Geometry: see drawing. Coordinates: mm, zero at the bounding-box minimum. A direction names the side the tool comes from. Give positions to 0.01 mm unless a question says otherwise; leave off trailing zeros. Write each loop counter-clockwise with the first axis right and the second up, starting at its lowest first coordinate (ties: lowest second). Pieces come first, ordered by that corner, then holes. Notation, with made-up numbers: (66, -11.5) -> (111, -11.5) arc R25 ccw to (111, 18.5) -> close; hole circle Ø1 at (-36, -17.5). An arc over 180 degrees is marked (long way). Use CSV: the item, a comma, the result in double quotes. Start each with the question number.
1) Contact query for flat-ended pins moving along their axis: P1, Ø5, axis at y = 376.5, z = 3.5, coming from the -X side; P2, Ø6, axis at x = 2, z = 17, coming from the +Y side; P3, Ø1, axis at x = 13, y = 163, coming from the -Z side; P4, Ø8, axis at y = 96.5, z = 5, coming from the +X side. Output: stop coordinate, or through.
2) Section A-A (z = 12.5). Output: boundary loops of the cut face in (x, y), plus the area to 3 significant figures.
3) Section B-B (y = 82). Output: boundary loops of the cut face in (x, z), plus the area to 3 significant figures.
4) Material intervals for line 1 (Y direction, x = 14.5, z = 11.75); line 2 (X direction, y = 422, z = 15); line 3 (Y direction, x = 18.75, z = 17) (1 decimal), sorted ascending. Write a range as [from, to].
5) Set-up query: the marked faces 1, 2 and 3. Return all of +Z, -Z, +X, -X, +Y, -Y with unobstructed straight access to the full face (end or side cutting, diameter ignored); none if empty.
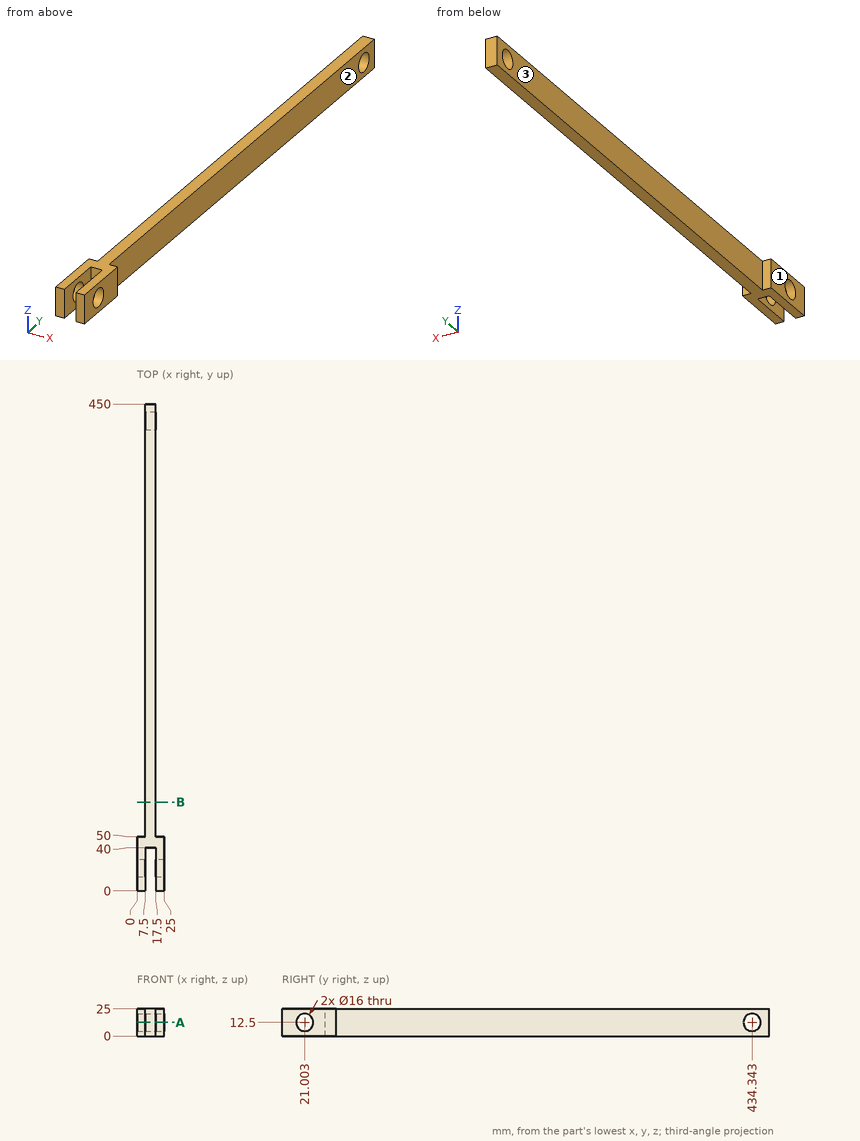
Answers follow:
1,P1,"stops at x = 7.5"
1,P2,"stops at y = 50"
1,P3,"stops at z = 0"
1,P4,"stops at x = 17.5"
2,outline,"(0, 0) -> (7.5, 0) -> (7.5, 13) -> (0, 13) -> close; (0, 29) -> (7.5, 29) -> (7.5, 40) -> (17.5, 40) -> (17.5, 29) -> (25, 29) -> (25, 50) -> (17.5, 50) -> (17.5, 426.34) -> (7.5, 426.34) -> (7.5, 50) -> (0, 50) -> close; (7.5, 442.34) -> (17.5, 442.34) -> (17.5, 450) -> (7.5, 450) -> close; (17.5, 0) -> (25, 0) -> (25, 13) -> (17.5, 13) -> close"
2,area,"4,450 mm^2"
3,outline,"(7.5, 0) -> (17.5, 0) -> (17.5, 25) -> (7.5, 25) -> close"
3,area,"250 mm^2"
4,line 1,"y = [40, 426.38], [442.31, 450]"
4,line 2,"x = [7.5, 17.5]"
4,line 3,"y = [0, 14.4], [27.6, 50]"
5,face 1,"+Z, -Z, -X, +Y, -Y"
5,face 2,"+Z, -Z, +X, +Y"
5,face 3,"+Z, -Z, -X, +Y"
